Could you check a few things on this drawing? It's one solid part, dimensions in mm from its lowest x, y, z. A direction names the side the tool comes from. Round coordinates to 2 decimals unless told otherwise and drop trailing zeros. Order: outer loops, then holes, each group sorted by start corner. A loop starts at its lowest first (then second) coordinate and runs counter-clockwise, first axis right, second up.
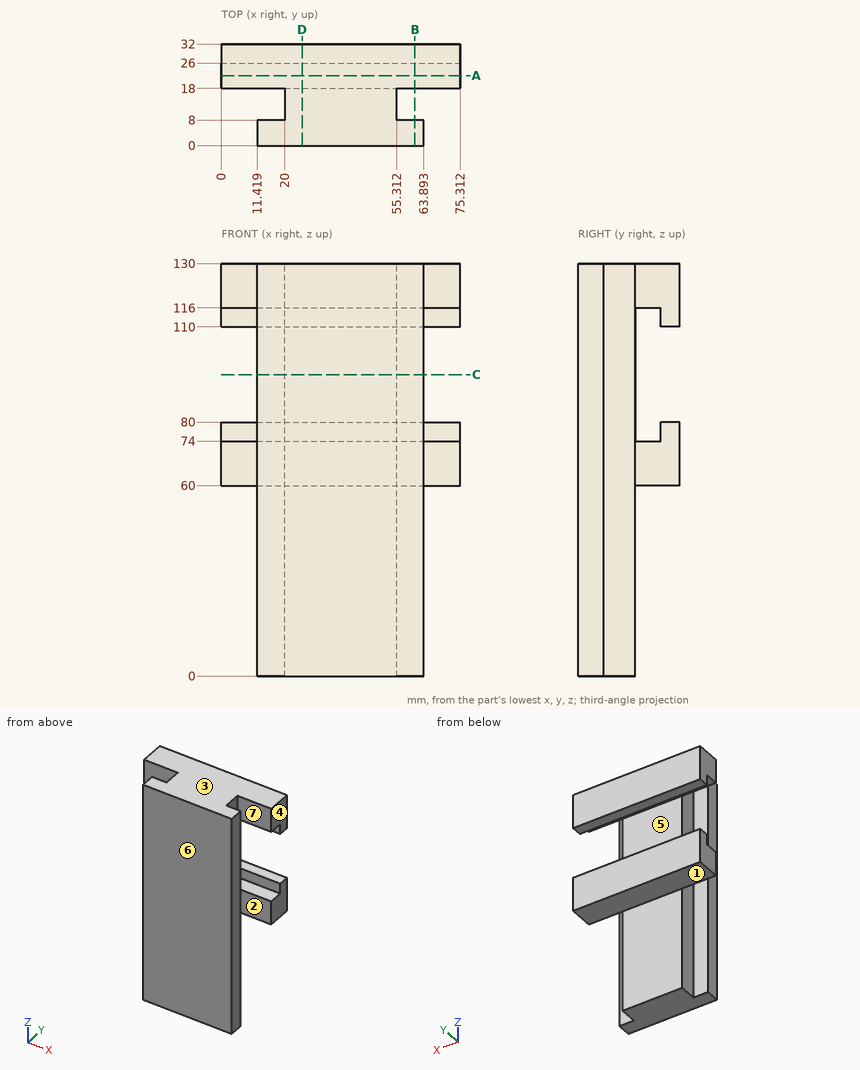
1) I'm going to push flat-ended pins straight in: pin 1 (9.5 mm diameter, centred on x = 59, z = 41.5, fed in from +Y); pin 2 (9 mm diameter, centred on y = 4.5, z = 61, fed in from -X); pin 3 (3 mm diameter, centred on y = 14, z = 50, fed in from -X); pin 4 (2 mm diameter, centred on x = 66.5, y = 9, fed in from +Z). Where does each tip first touch, or does it pass through?
2) If we section it at C-C (z = 95): Write out the boundary of the cut face in (x, y).
3) If we section it at B-B (x = 61): Write out the boundary of the cut face in (y, z).
4) If we section it at D-D (x = 25.5): Write out the boundary of the cut face in (y, z), plus the area to 3 significant figures.
5) For the marked faces 1, 2 and 3, which set-ups out of +Z, -Z, +X, -X, +Y, -Y let a thin tool reach every point of the face, with its end or its side?
6) If we section it at A-A (y = 22): Write out the boundary of the cut face in (x, z), plus the area to 3 significant figures.
7) I need wall thicknesses on line 1 (Z direction, x = 51.5, y = 30); line 2 (Y direction, x = 13.5, z = 113); line 3 (Y direction, x = 56.5, z = 69). Which ranges of each line are inside material? Lowest first, please.
8) We'd pull the mould along Y, two halves only. Please class the marked faces 4, 5, 6 and 7: +Y half, -Y half, draft (parallel to the pull), parting line (faces both ways), or undercut.
Solutions:
1. pin 1: stops at y = 18
1. pin 2: stops at x = 11.42
1. pin 3: stops at x = 20
1. pin 4: passes through
2. outline: (11.42, 0) - (63.89, 0) - (63.89, 8) - (55.31, 8) - (55.31, 18) - (20, 18) - (20, 8) - (11.42, 8) - close
3. outline: (0, 0) - (8, 0) - (8, 130) - (0, 130) - close; (18, 60) - (32, 60) - (32, 80) - (26, 80) - (26, 74) - (18, 74) - close; (18, 116) - (26, 116) - (26, 110) - (32, 110) - (32, 130) - (18, 130) - close
4. outline: (0, 0) - (18, 0) - (18, 60) - (32, 60) - (32, 80) - (26, 80) - (26, 74) - (18, 74) - (18, 116) - (26, 116) - (26, 110) - (32, 110) - (32, 130) - (0, 130) - close
4. area: 2,800 mm2
5. face 1: -Z, +X, -X, +Y
5. face 2: +Z, -Z, +X
5. face 3: +Z, +X, -X, +Y, -Y
6. outline: (0, 60) - (75.31, 60) - (75.31, 74) - (0, 74) - close; (0, 116) - (75.31, 116) - (75.31, 130) - (0, 130) - close
6. area: 2,110 mm2
7. line 1: z = 60 to 80, 110 to 130
7. line 2: y = 0 to 8, 26 to 32
7. line 3: y = 0 to 8, 18 to 32
8. face 4: draft
8. face 5: undercut
8. face 6: -Y half
8. face 7: undercut
